Autodesk Inventor part; units mm, degrees
ref_plane "YZ Plane" through (0, 0, 0) normal (1, 0, 0) x (0, 1, 0)
ref_plane "XZ Plane" through (0, 0, 0) normal (0, 1, 0) x (-1, 0, 0)
ref_plane "XY Plane" through (0, 0, 0) normal (0, 0, 1) x (1, 0, 0)
sketch "Sketch1" plane through (0, 0, 0) normal (1, 0, 0) x (0, 1, 0)
  circle A0 centre (0, 0) radius 18
  dimension "d0" = 36
extrude "Extrusion1" add sketch "Sketch1" along normal blind 173
sketch "Sketch2" plane through (0, 0, 0) normal (-1, 0, 0) x (0, 0, 1)
  line L0 (20, -8) -> (-20, -8)
  line L1 (-20, -8) -> (-20, 8)
  line L2 (-20, 8) -> (20, 8)
  line L3 (20, 8) -> (20, -8)
  line L4 (20, -8) -> (-20, 8) construction
  line L5 (-20, -8) -> (20, 8) construction
  circle A0 centre (0, 0) radius 18
  arc A1 (-16.1245, -8) -> (-17.098, -5.6266) centre (0, 0) ccw
  dimension "d3" = 40
  dimension "d5" = 16
extrude "Extrusion2" add sketch "Sketch2" along normal blind 27 contours A0 L2 L0 | L0 L1 L2 A0 | A0 L2 L3 L0
sketch "Sketch3" plane through (-27, 0, 0) normal (-1, 0, 0) x (0, 0, 1)
  circle A0 centre (0, 0) radius 18
  circle A1 centre (0, 0) radius 50
  dimension "d8" = 36
  dimension "d9" = 100
extrude "Extrusion3" cut sketch "Sketch3" against normal blind 27
sketch "Sketch4" plane through (0, 8, 16.1245) normal (0, 1, 0) x (1, 0, 0)
  circle A0 centre (-15, 16.1245) radius 5
  line L0 (-27, 0) -> (0, 0)
  line L1 (-27, 0) -> (-27, 32.249)
  point P0 (0, 16.1245)
  dimension "d12" = 10
  dimension "d13" = 16.1245
  dimension "d14" = 12
extrude "Extrusion4" cut sketch "Sketch4" against normal blind 16
properties part number "MSAL 32 50 Stand In"
Verification items for the finished model (mm, model axes). A direction names the side the tool comes from. Give positions to 0.01 mm unless a question says otherwise; leave off trailing zeros. Write each loop counter-clockwise with the first axis right and the second up, starting at its lowest first coordinate (ties: lowest second). Pieces come first, ordered by that corner, then holes. Notation, with made-up numbers: (85, 81) - (129, 81) arc R38 ccw to (129, 119) - close; hole circle Ø7 at (29.5, 23). An arc over 180 degrees is marked (long way). Put each result on its own line as item: value.
Q1. Section check B-B on z = 0. Record the cut outline in (x, y), and give its area (3 significant figures).
Result:
outline: (-27, -8) - (-20, -8) - (-20, 8) - (-27, 8) - close; (-10, -8) - (0, -8) - (0, -18) - (173, -18) - (173, 18) - (0, 18) - (0, 8) - (-10, 8) - close
area: 6,500 mm2
Q2. Section check A-A on x = -15. Record the cut outline in (y, z).
Result:
outline: (-8, -16.12) arc R18 ccw to (8, -16.12) - (8, -5) - (-8, -5) - close; (-8, 5) - (8, 5) - (8, 16.12) arc R18 ccw to (-8, 16.12) - close
Q3. Depth check by flat-ended pin: P1, Ø21.5, axis at x = -15.5, z = -6, coming from the +Y side; P2, Ø3, axis at x = 112.5, y = -6, coming from the +Z side; P3, Ø3, axis at y = 11.5, z = 9.5, coming from the -X side. Enter the tip coordinate at first touch or a pass-through.
Result:
P1: y = 8
P2: z = 17.43
P3: x = 0
Q4. Section check D-D on x = 49. Record the cut outline in (y, z).
Result:
outline: circle Ø36 at (0, 0)
Q5. Scan lines: probe 1 along Z at (x, y) = (-15, 0); probe 2 along X at (y, z) = (0, 0); probe 3 along Z at (x, y) = (-15, -3.5). Record each from-to range of solid material in increasing order. Write a range as from..to.
Result:
probe 1: -18..-5, 5..18
probe 2: -27..-20, -10..173
probe 3: -17.66..-5, 5..17.66
Q6. Set-up check for faces 3 (the face through (173, 0, 0)), 4 (the face through (0, -12, 0)), 5 (the face through (-10, 8, 3)): record each of +Z, -Z, +X, -X, +Y, -Y from which the full face is reachable in a straight line by a thin tool's end or side.
Result:
face 3: +Z, -Z, +X, +Y, -Y
face 4: +Z, -Z, -X, -Y
face 5: +Z, -Z, -X, +Y
Q7. Mould release check, pull along Z, two halves, no side actions. Record for faces 1 (the face through (-20, 0, 0)), 2 (the face through (0, 12, 0)): released by +Z, released by -Z, zero draft, split by the parting line, or undercut.
Result:
face 1: undercut
face 2: zero draft
Q8. Section check C-C on y = 3. Record the cut outline in (x, z), and give its area (3 significant figures).
Result:
outline: (-27, -17.75) - (173, -17.75) - (173, 17.75) - (-27, 17.75) - close; hole circle Ø10 at (-15, 0)
area: 7,020 mm2
